The drawing under review shows one solid part. Ordinate dimensions are in mm from its lowest x, y, z. A direction names the side the tool comes from. Give positions to 0.01 mm unless a question says otherwise; leave off trailing zeros. Loops run counter-clockwise (first coordinate to the right, second up) from the corner with the lowest first, then second, coordinate; pieces in that order, holes last.
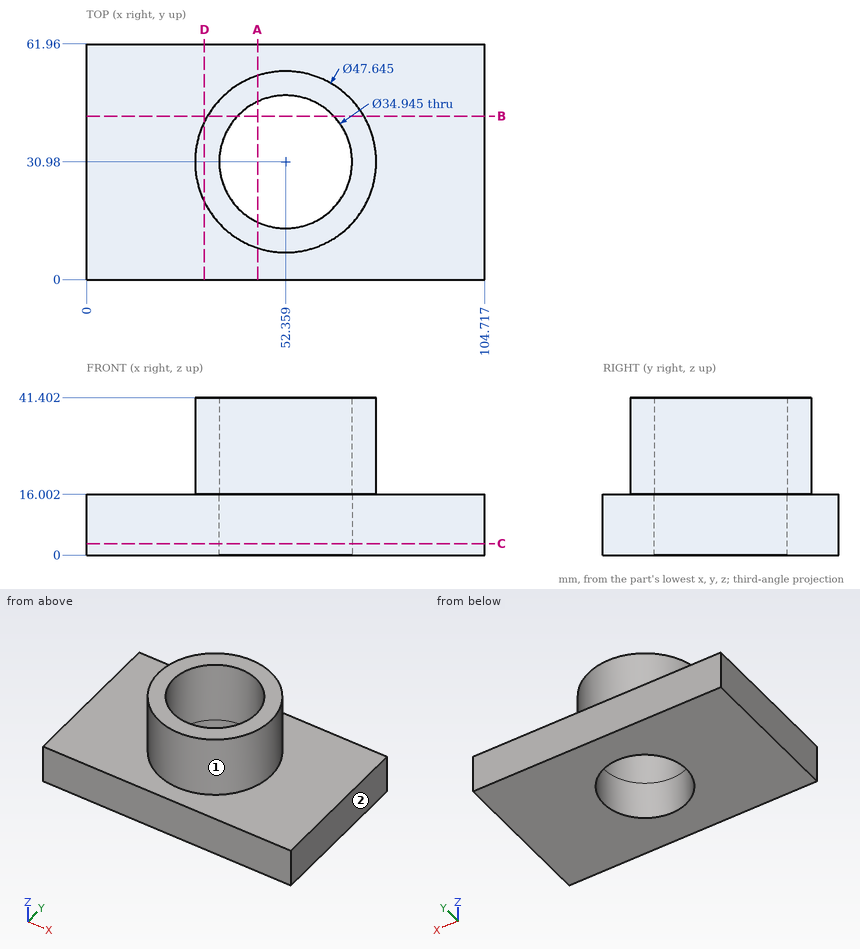
Item 1: Take a section at C-C on z = 3. Give the boundary of the cut face in (x, y) (1 decimal), and give its area (3 significant figures).
Answer:
outline: (0, 0) - (104.7, 0) - (104.7, 62) - (0, 62) - close; hole circle Ø34.9 at (52.4, 31)
area: 5,530 mm2
Item 2: For L1, parallel to Z at x = 96.5, y = 18; L2, parallel to Y at x = 67, z = 26 (1 decimal); L3, parallel to X at y = 22.5, z = 14.5 (1 decimal), list the stretches that pass through material, from the lowest coordinate up.
Answer:
L1: z = 0 to 16
L2: y = 12.2 to 21.4, 40.5 to 49.8
L3: x = 0 to 37.1, 67.6 to 104.7
Item 3: Tool access review of the marked faces 1 and 2: name each direction out of +Z, -Z, +X, -X, +Y, -Y from which nothing blocks a thin tool from reaching the whole face with its end or side.
Answer:
face 1: +Z
face 2: +Z, -Z, +X, +Y, -Y
Item 4: Clearance check with flat-ended pins moving along their axes: pin 1 Ø4 at (x, y) = (90.5, 6) entering from +Z; pin 2 Ø5 at (x, z) = (46, 25.5) entering from +Y. State where each tip first meets the part, or that it passes through.
Answer:
pin 1: stops at z = 16
pin 2: stops at y = 54.49
Item 5: Take a section at B-B on y = 43. Give the boundary of the cut face in (x, z).
Answer:
outline: (0, 0) - (39.68, 0) - (39.68, 41.4) - (31.79, 41.4) - (31.79, 16) - (0, 16) - close; (65.04, 0) - (104.72, 0) - (104.72, 16) - (72.93, 16) - (72.93, 41.4) - (65.04, 41.4) - close
Item 6: Take a section at A-A on x = 45. Give the boundary of the cut face in (y, z).
Answer:
outline: (0, 0) - (15.13, 0) - (15.13, 41.4) - (8.32, 41.4) - (8.32, 16) - (0, 16) - close; (46.83, 0) - (61.96, 0) - (61.96, 16) - (53.64, 16) - (53.64, 41.4) - (46.83, 41.4) - close
Item 7: Take a section at D-D on x = 31. Give the boundary of the cut face in (y, z), and give its area (3 significant figures).
Answer:
outline: (0, 0) - (61.96, 0) - (61.96, 16) - (41.53, 16) - (41.53, 41.4) - (20.43, 41.4) - (20.43, 16) - (0, 16) - close
area: 1,530 mm2
